Check sheet for the modelled part. Datum: model origin and axes. Units: mm. Face numbers are marked on the shaded views. Coordinates: 2 decimals unless noted, no trailing zeros. Order: outer loops, then holes, each group sorted by start corner. A loop starts at its lowest first (then second) coordinate and runs counter-clockwise, first axis right, second up.
Autodesk Inventor part; units mm, degrees
ref_plane "YZ Plane" through (0, 0, 0) normal (1, 0, 0) x (0, 1, 0)
ref_plane "XZ Plane" through (0, 0, 0) normal (0, 1, 0) x (-1, 0, 0)
ref_plane "XY Plane" through (0, 0, 0) normal (0, 0, 1) x (1, 0, 0)
sketch "Sketch1" plane through (0, 0, 0) normal (0, 0, 1) x (1, 0, 0)
  line L0 (100, 0.14) -> (100, 0)
  line L1 (0, 0.14) -> (0, 0)
  arc A0 (96.9975, 0) -> (94, 4) centre (93.0167, 0.14) ccw
  arc A1 (100, 0.14) -> (94.323, 7) centre (93.0167, 0.14) ccw
  arc A2 (6, 4) -> (3.0025, 0) centre (6.9833, 0.14) ccw
  arc A3 (5.677, 7) -> (0, 0.14) centre (6.9833, 0.14) ccw
  line L2 (5.677, 7) -> (94.323, 7)
  line L3 (96.9975, 0) -> (100, 0)
  line L4 (6, 4) -> (94, 4)
  line L5 (3, 0.14) -> (3, 0)
  line L6 (0, 0) -> (3.0025, 0)
  dimension "d0" = 100
  dimension "d6" = 3
  dimension "d7" = 7
  dimension "d8" = 3
extrude "Extrusion1" add sketch "Sketch1" along normal blind 14
sketch "Sketch2" plane through (5.677, 7, 0) normal (0, 1, 0) x (1, 0, 0)
  line L0 (0, -14) -> (88.6461, -14)
  line L1 (0, 0) -> (88.6461, 0)
  line L2 (44.323, 0) -> (44.323, -14)
  point P0 (-5.677, 0)
  point P1 (14.323, -7)
  point P2 (33.323, -7)
  point P3 (55.323, -7)
  point P4 (74.323, -7)
  dimension "d11" = 22
  dimension "d12" = 60
  dimension "d13" = 11
  dimension "d14" = 30
  dimension "d15" = 7
hole "Hole1" at (20, 7, 7) at (39, 7, 7) at (61, 7, 7) at (80, 7, 7) direction (0, -1, 0) diameter 3.2 depth 3 tip angle 118
properties part number "LAMINA"
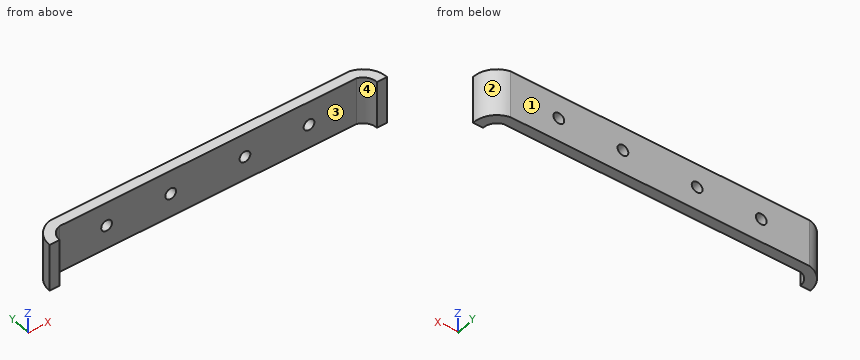
(1) Cross-section at A-A (x = 61). Enter the section's corners in (y, z).
Filled in:
outline: (4, 0) - (7, 0) - (7, 5.4) - (4, 5.4) - close; (4, 8.6) - (7, 8.6) - (7, 14) - (4, 14) - close
(2) Thickness scan on probe 1 along Z at (x, y) = (20, 5); probe 2 along X at (y, z) = (5.3, 7); probe 3 along X at (y, z) = (6.45, 7). Record the ranges inside material, lowest first.
Filled in:
probe 1: z = 0 to 5.4, 8.6 to 14
probe 2: x = 2.28 to 18.4, 21.6 to 37.4, 40.6 to 59.4, 62.6 to 78.4, 81.6 to 97.72
probe 3: x = 3.99 to 18.4, 21.6 to 37.4, 40.6 to 59.4, 62.6 to 78.4, 81.6 to 96.01
(3) Release check for a two-part mould opening along X. For the marked faces 1, 2, 3 and 4 record: +X half, -X half, draft (parallel to the pull), parting line (faces both ways), or undercut.
Filled in:
face 1: draft
face 2: +X half
face 3: undercut
face 4: undercut
(4) Cross-section at D-D (z = 11). Enter the section's corners in (x, y), and give its area (3 significant figures).
Filled in:
outline: (0, 0) - (3, 0) arc R3.98 cw to (6, 4) - (94, 4) arc R3.98 cw to (97, 0) - (100, 0) - (100, 0.14) arc R6.98 ccw to (94.32, 7) - (5.68, 7) arc R6.98 ccw to (0, 0.14) - close
area: 311 mm2
(5) Cross-section at B-B (y = 2.25). Enter the section's corners in (x, z), and give its area (3 significant figures).
Filled in:
outline: (0.33, 0) - (3.6, 0) - (3.6, 14) - (0.33, 14) - close; (96.4, 0) - (99.67, 0) - (99.67, 14) - (96.4, 14) - close
area: 91.8 mm2
(6) Cross-section at C-C (z = 7.25). Enter the section's corners in (x, y), and give its area (3 significant figures).
Filled in:
outline: (0, 0) - (3, 0) arc R3.98 cw to (6, 4) - (18.42, 4) - (18.42, 7) - (5.68, 7) arc R6.98 ccw to (0, 0.14) - close; (21.58, 4) - (37.42, 4) - (37.42, 7) - (21.58, 7) - close; (40.58, 4) - (59.42, 4) - (59.42, 7) - (40.58, 7) - close; (62.58, 4) - (78.42, 4) - (78.42, 7) - (62.58, 7) - close; (81.58, 4) - (94, 4) arc R3.98 cw to (97, 0) - (100, 0) - (100, 0.14) arc R6.98 ccw to (94.32, 7) - (81.58, 7) - close
area: 273 mm2
(7) Go/stop test with flat-tipped pins: P1, Ø2, axis at y = 5, z = 4, coming from the -X side; P2, Ø1, axis at y = 1, z = 4.5, coming from the +X side. Record where each tip stops, or that it passes through.
Filled in:
P1: stops at x = 1.16
P2: stops at x = 99.99
